from build123d import *

# Parameters (mm, degrees)
SKETCH1_W           = 86.36
SKETCH1_H           = 2.54
BOSS_EXTRUDE1_DEPTH = 149.86
SKETCH2_W           = 86.36
SKETCH2_H           = 2.54
BOSS_EXTRUDE2_DEPTH = 38.1
SKETCH3_R           = 6.096
CUT_EXTRUDE1_DEPTH  = 41.64


with BuildPart() as part:
    # Sketch1 → Boss-Extrude1 (new body)
    with BuildSketch(Plane(origin=(0, 0, 0), x_dir=(1, 0, 0), z_dir=(0, 1, 0))):
        Rectangle(SKETCH1_W, SKETCH1_H)
    extrude(amount=BOSS_EXTRUDE1_DEPTH)

    # Sketch2 → Boss-Extrude2 (add)
    with BuildSketch(Plane(origin=(0, 0, -1.27), x_dir=(-1, 0, 0), z_dir=(0, 0, -1))):
        with Locations((0, 148.59)):
            Rectangle(SKETCH2_W, SKETCH2_H)
    extrude(amount=BOSS_EXTRUDE2_DEPTH)

    # Sketch3 → Cut-Extrude1 (cut, through all)
    with BuildSketch(Plane.XY.offset(1.27)):
        with Locations((0, 129.655411205)):
            Circle(SKETCH3_R)
        with Locations((0, 91.555411205)):
            Circle(SKETCH3_R)
        with Locations((0, 53.455411205)):
            Circle(SKETCH3_R)
    extrude(amount=-CUT_EXTRUDE1_DEPTH, mode=Mode.SUBTRACT)


solid = part.part
Build history of the part. All positions in model axes, mm. A direction names the side the tool comes from. Round coordinates to 2 decimals unless told otherwise and drop trailing zeros. Order: outer loops, then holes, each group sorted by start corner. A loop starts at its lowest first (then second) coordinate and runs counter-clockwise, first axis right, second up. Notation, with made-up numbers: M 15.5,18 L 55.5,18 A13 cw 55.5,32 Z; hole C 45,13 d7. An arc over 180 degrees is marked long. Use CSV: the item, a comma, the result in double quotes. Start each with the question number.
(1) Tool access for faces 1 (the face through (43.18, 75, 1)), 2 (the face through (1, 147.32, -20)): list every direction of +Z, -Z, +X, -X, +Y, -Y with a clear straight run to the whole face (end or side of a thin tool).
(2) Cut at B-B on y = 128. List the corners of the cut face in (x, z).
(3) Cut at D-D on y = 39. List the corners of the cut face in (x, z), then the cut area to 3 significant figures.
(4) Cut at C-C on z = -14. List the corners of the cut face in (x, y).
(5) Cut at A-A on x = 0. List the corners of the cut face in (y, z), then the cut area to 3 significant figures.
(6) Drill centre lines: probe 1 along Y at (x, z) = (0, 0.25); probe 2 along Z at (x, y) = (20, 53.5); probe 3 along Y at (x, z) = (-11, -6.5). Where is each one in solid material? Low to high.
(7) Flat gauge pins, fed straight in: P1, Ø6, axis at x = 16.5, z = -10, coming from the -Y side; P2, Ø14, axis at x = 0, y = 53.46, coming from the +Z side. Where does each tip first touch, or does it go through?
(8) Mould opens along X. For faces 3 (the face through (1, 149.86, -19)), 4 (the face through (3.277, 58.596, 0.018)), 5 (the face through (-43.18, 75, 1)) say: +X half, -X half, draft (parallel to the pull), parting line (faces both ways), or undercut.
Findings:
1,face 1,"+Z, -Z, +X, +Y, -Y"
1,face 2,"-Z, +X, -X, -Y"
2,outline,"M -43.18,-1.27 L -5.87,-1.27 L -5.87,1.27 L -43.18,1.27 Z; M 5.87,-1.27 L 43.18,-1.27 L 43.18,1.27 L 5.87,1.27 Z"
3,outline,"M -43.18,-1.27 L 43.18,-1.27 L 43.18,1.27 L -43.18,1.27 Z"
3,area,"219 mm^2"
4,outline,"M -43.18,147.32 L 43.18,147.32 L 43.18,149.86 L -43.18,149.86 Z"
5,outline,"M 0,-1.27 L 47.36,-1.27 L 47.36,1.27 L 0,1.27 Z; M 59.55,-1.27 L 85.46,-1.27 L 85.46,1.27 L 59.55,1.27 Z; M 97.65,-1.27 L 123.56,-1.27 L 123.56,1.27 L 97.65,1.27 Z; M 135.75,-1.27 L 147.32,-1.27 L 147.32,-39.37 L 149.86,-39.37 L 149.86,1.27 L 135.75,1.27 Z"
5,area,"385 mm^2"
6,probe 1,"y = 0 to 47.36, 59.55 to 85.46, 97.65 to 123.56, 135.75 to 149.86"
6,probe 2,"z = -1.27 to 1.27"
6,probe 3,"y = 147.32 to 149.86"
7,P1,"stops at y = 147.32"
7,P2,"stops at z = 1.27"
8,face 3,"draft"
8,face 4,"undercut"
8,face 5,"-X half"
